from build123d import *

# Parameters (mm, degrees)
F1_DEPTH = 170.18
F2_W     = 49.288719
F2_H     = 32.279059
F3_DEPTH = 25.4


with BuildPart() as f1:
    # F0 (on Front) → F1 (new body)
    with BuildSketch(Plane.XZ):
        with BuildLine():
            Line((-9.986188, 0), (0, 0))
            Line((0, 0), (114.473812, 0))
            ThreePointArc((114.473812, 0), (116.269863, 0.743949), (117.013812, 2.54))
            Line((117.013812, 2.54), (117.013812, 100.33))
            Line((117.013812, 100.33), (115.743812, 100.33))
            Line((115.743812, 100.33), (115.743812, 3.81))
            ThreePointArc((115.743812, 3.81), (114.999863, 2.013949), (113.203812, 1.27))
            Line((113.203812, 1.27), (-8.716188, 1.27))
            ThreePointArc((-8.716188, 1.27), (-10.512239, 2.013949), (-11.256188, 3.81))
            Line((-11.256188, 3.81), (-11.256188, 52.07))
            Line((-11.256188, 52.07), (-12.526188, 52.07))
            Line((-12.526188, 52.07), (-12.526188, 2.54))
            ThreePointArc((-12.526188, 2.54), (-11.782239, 0.743949), (-9.986188, 0))
        make_face()
    extrude(amount=-F1_DEPTH)

    # F2 (on face) → F3 (cut)
    with BuildSketch(Plane.XY.offset(1.27)):
        with Locations((32.944252, 99.213123)):
            Rectangle(F2_W, F2_H)
    extrude(amount=-F3_DEPTH, mode=Mode.SUBTRACT)


solid = f1.part
Model file for the job. Use its own axes, mm. A direction names the side the tool comes from. Give positions to 0.01 mm unless a question says otherwise; leave off trailing zeros. Write each loop counter-clockwise with the first axis right and the second up, starting at its lowest first coordinate (ties: lowest second). Pieces come first, ordered by that corner, then holes. Notation, with made-up numbers: (27, 45.5) -> (46, 45.5) arc R29 cw to (46, 75.5) -> close; hole circle Ø9 at (1.5, 35). An arc over 180 degrees is marked (long way). Write item = value, one per line.
(1) Slice it at D-D, the plane x = 94. Give the cut face in (y, z), then the cut area to 3 significant figures.
Determined:
outline = (0, 0) -> (170.18, 0) -> (170.18, 1.27) -> (0, 1.27) -> close
area = 216 mm2
(2) Mould opens along X. For faces 1 (the face through (117.014, 84, 51)), 2 (the face through (115.744, 84, 53)), 3 (the face through (65, 84, 0)) say: released by +X, released by -X, zero draft, split by the parting line, or undercut.
Determined:
face_1 = released by +X
face_2 = undercut
face_3 = zero draft
(3) Tool access for faces 4 (the face through (-12.526, 84, 28)), 5 (the face through (67, 84, 1.27)): list every direction of +Z, -Z, +X, -X, +Y, -Y with a clear straight run to the whole face (end or side of a thin tool).
Determined:
face_4 = +Z, -Z, -X, +Y, -Y
face_5 = +Z, +Y, -Y
(4) Probe line 1 along X through (y, z) = (23, 37); line 2 along Z through (x, y) = (90.5, 77.5); line 3 along X through (y, z) = (156.5, 59.5). List the from-to ranges inside material, lowest first.
Determined:
line_1 = -12.53 to -11.26, 115.74 to 117.01
line_2 = 0 to 1.27
line_3 = 115.74 to 117.01
(5) Slice it at A-A, the plane z = 32. Give the cut face in (x, y).
Determined:
outline = (-12.53, 0) -> (-11.26, 0) -> (-11.26, 170.18) -> (-12.53, 170.18) -> close; (115.74, 0) -> (117.01, 0) -> (117.01, 170.18) -> (115.74, 170.18) -> close
(6) Slice it at B-B, the plane x = 41. Give the cut face in (y, z).
Determined:
outline = (0, 0) -> (83.07, 0) -> (83.07, 1.27) -> (0, 1.27) -> close; (115.35, 0) -> (170.18, 0) -> (170.18, 1.27) -> (115.35, 1.27) -> close
(7) Slice it at C-C, the plane y = 34. Give the cut face in (x, z).
Determined:
outline = (-12.53, 2.54) arc R2.54 ccw to (-9.99, 0) -> (114.47, 0) arc R2.54 ccw to (117.01, 2.54) -> (117.01, 100.33) -> (115.74, 100.33) -> (115.74, 3.81) arc R2.54 cw to (113.2, 1.27) -> (-8.72, 1.27) arc R2.54 cw to (-11.26, 3.81) -> (-11.26, 52.07) -> (-12.53, 52.07) -> close
(8) Flat gauge pins, fed straight in: P1, Ø8, axis at x = 43, y = 84, coming from the -Z side; P2, Ø1, axis at x = -12, y = 58.5, coming from the +Z side; P3, Ø10, axis at x = 87.5, y = 72.5, coming from the +Z side; P4, Ø1.4, axis at y = 99.5, z = 0.5, coming from the +X side. Where does each tip first touch, or does it go through?
Determined:
P1 = 0
P2 = 52.07
P3 = 1.27
P4 = 116.63
